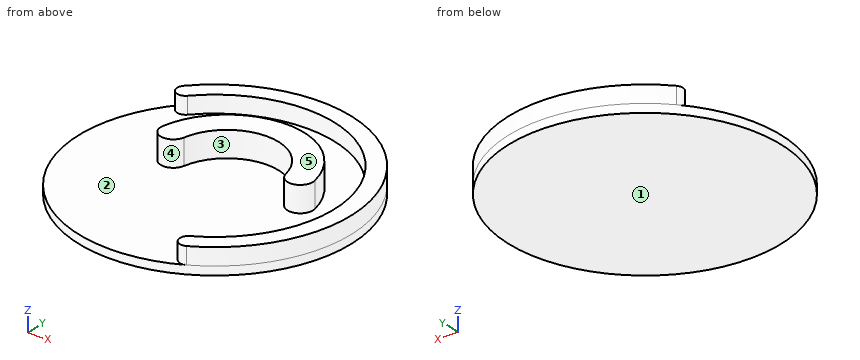
from build123d import *

# Parameters (mm, degrees)
SKETCH1_R           = 16
BOSS_EXTRUDE1_DEPTH = 1
BOSS_EXTRUDE2_DEPTH = 3
BOSS_EXTRUDE3_START = 2
BOSS_EXTRUDE3_DEPTH = 2


with BuildPart() as part:
    # Sketch1 → Boss-Extrude1 (new body)
    with BuildSketch(Plane.XY):
        with Locations((24.677925359, 4)):
            Circle(SKETCH1_R)
    extrude(amount=-BOSS_EXTRUDE1_DEPTH)

    # Sketch1<3> → Boss-Extrude2 (add)
    with BuildSketch(Plane.XY):
        with BuildLine():
            ThreePointArc((34.952555431, 5.797906435), (26.080180575, 13.052706951), (17.207805718, 5.797906435))
            ThreePointArc((17.207805718, 5.797906435), (18.380018924, 4.02988036), (20.148044999, 5.202093565))
            ThreePointArc((20.148044999, 5.202093565), (26.080180575, 10.052706951), (32.01231615, 5.202093565))
            ThreePointArc((32.01231615, 5.202093565), (33.780342225, 4.02988036), (34.952555431, 5.797906435))
        make_face()
    extrude(amount=BOSS_EXTRUDE2_DEPTH)

    # Sketch2 → Boss-Extrude3 (add)
    with BuildSketch(Plane.XY.offset(BOSS_EXTRUDE3_START)):
        with BuildLine():
            ThreePointArc((32.111206734, -10.168497733), (37.340396009, 13.78068694), (12.847014077, 14.771700806))
            ThreePointArc((12.847014077, 14.771700806), (12.913214732, 13.35903755), (14.325877987, 13.425238205))
            ThreePointArc((14.325877987, 13.425238205), (35.757587178, 12.558101073), (31.182046562, -8.397435516))
            ThreePointArc((31.182046562, -8.397435516), (30.761095539, -9.74754671), (32.111206734, -10.168497733))
        make_face()
    extrude(amount=-BOSS_EXTRUDE3_DEPTH)


solid = part.part
Source: CAD feature listing. Evaluate the final solid. Frame: model axes, mm. Face numbers are marked on the shaded views. A direction names the side the tool comes from. Coordinates: 2 decimals unless noted, no trailing zeros. Order: outer loops, then holes, each group sorted by start corner. A loop starts at its lowest first (then second) coordinate and runs counter-clockwise, first axis right, second up.
Item 1: Cut plane C-C (y = 7.5). Return loops of the section in (x, z), plus the area to 3 significant figures.
Output values:
outline: (9.07, -1) - (40.29, -1) - (40.29, 2) - (38.23, 2) - (38.23, 0) - (34.43, 0) - (34.43, 3) - (31.02, 3) - (31.02, 0) - (21.14, 0) - (21.14, 3) - (17.73, 3) - (17.73, 0) - (9.07, 0) - close
area: 55.8 mm2
Item 2: Material intervals for line 1 (Z direction, x = 38, y = 11.5); line 2 (Y direction, x = 32.5, z = 0.45); line 3 (Y direction, x = 24.5, z = -0.5), sorted ascending.
Output values:
line 1: z = -1 to 2
line 2: y = -9.96 to -7.61, 4.37 to 10.38, 15.61 to 17.96
line 3: y = -12 to 20
Item 3: Set-up query: the marked faces 1 and 2. Return all of +Z, -Z, +X, -X, +Y, -Y with unobstructed straight access to the full face (end or side cutting, diameter ignored); none if empty.
Output values:
face 1: -Z, +X, -X, +Y, -Y
face 2: +Z
Item 4: Cut plane D-D (x = 36.5). Return loops of the section in (y, z), plus the area to 3 significant figures.
Output values:
outline: (-6.78, -1) - (14.78, -1) - (14.78, 2) - (11.5, 2) - (11.5, 0) - (-3.5, 0) - (-3.5, 2) - (-6.78, 2) - close
area: 34.7 mm2
Item 5: First-contact query: P1, Ø1.5, axis at y = -4.5, z = 0, coming from the -X side; P2, Ø1, axis at x = 25.5, y = -1, coming from the +Z side. Flat tips, straight axial feed; report the tip coordinate or a pass-through.
Output values:
P1: stops at x = 10.68
P2: stops at z = 0
Item 6: Pull-direction query (X, two-part tool) for the marked faces 3, 4 and 5; classes: pulls with the +X half, pulls with the -X half, needs draft (parallel to the pull), parting line crosses it, or undercut.
Output values:
face 3: undercut
face 4: undercut
face 5: needs draft
Item 7: Cut plane B-B (x = 25). Return loops of the section in (y, z), plus the area to 3 significant figures.
Output values:
outline: (-12, -1) - (20, -1) - (20, 2) - (18, 2) - (18, 0) - (12.99, 0) - (12.99, 3) - (9.96, 3) - (9.96, 0) - (-12, 0) - close
area: 45.1 mm2
Item 8: Cut plane A-A (z = 1.25). Return loops of the section in (x, y), plus the area to 3 significant figures.
Output values:
outline: (12.85, 14.77) arc R1 ccw to (14.33, 13.43) arc R14 cw (long way) to (31.18, -8.4) arc R1 ccw to (32.11, -10.17) arc R16 ccw (long way) to start; (17.21, 5.8) arc R1.5 ccw to (20.15, 5.2) arc R6.05 cw to (32.01, 5.2) arc R1.5 ccw to (34.95, 5.8) arc R9.05 ccw to start
area: 177 mm2
